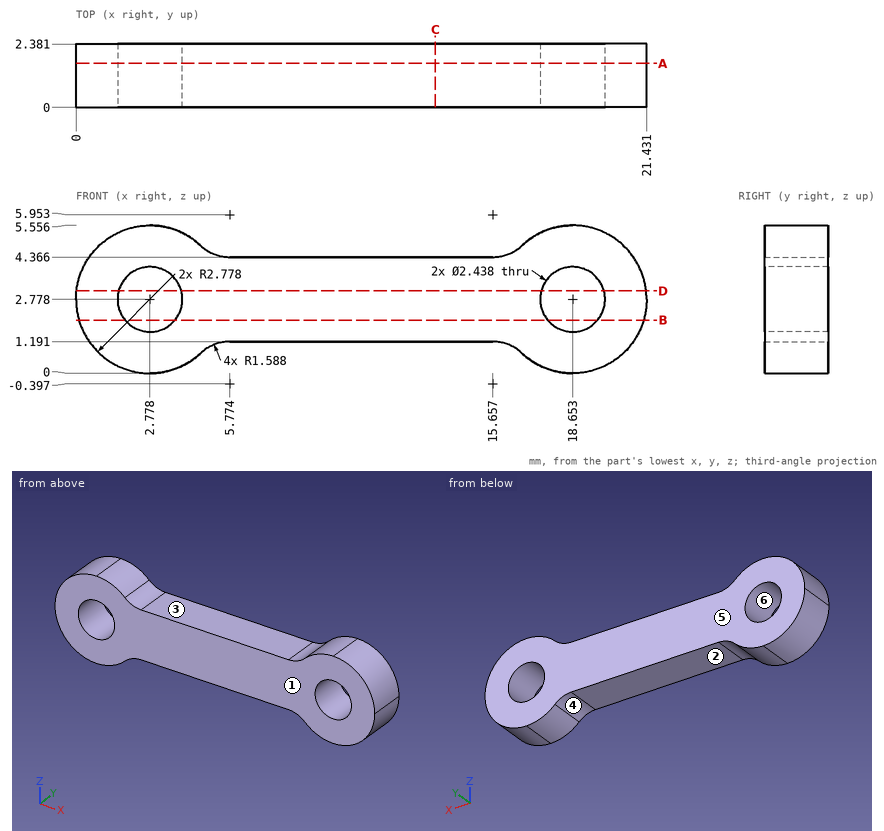
Source: three-view drawing plus pictorial views. Frame: mm from the lowest corner of the part. A direction names the side the tool comes from. Round coordinates to 2 decimals unless told otherwise and drop trailing zeros. Order: outer loops, then holes, each group sorted by start corner. A loop starts at its lowest first (then second) coordinate and runs counter-clockwise, first axis right, second up. Notation, with made-up numbers: M -39.75,-18.75 L 12.25,-18.75 A32 ccw 12.25,20.25 Z; hole C 50.5,-13 d1. An arc over 180 degrees is marked long. One line per item, written item: value.
(1) Cut plane C-C (x = 13.5). Return the cut outline in (y, z) (1 decimal).
Result sheet:
outline: M 0,1.2 L 2.4,1.2 L 2.4,4.4 L 0,4.4 Z
(2) Cut plane B-B (z = 2). Return the cut outline in (x, y) (1 decimal).
Result sheet:
outline: M 0.1,0 L 1.8,0 L 1.8,2.4 L 0.1,2.4 Z; M 3.7,0 L 17.7,0 L 17.7,2.4 L 3.7,2.4 Z; M 19.6,0 L 21.3,0 L 21.3,2.4 L 19.6,2.4 Z
(3) Pin query (flat end, axial travel): P1, Ø0.7, axis at x = 12.5, y = 1, coming from the -Z side; P2, Ø1.2, axis at x = 8.5, y = 1.5, coming from the +Z side. Return the tip coordinate at first contact, or that it passes through.
Result sheet:
P1: z = 1.19
P2: z = 4.37
(4) Pull-direction query (Z, two-part tool) for the marked faces 4, 5 and 6; classes: pulls with the +Z half, pulls with the -Z half, needs draft (parallel to the pull), parting line crosses it, or undercut.
Result sheet:
face 4: pulls with the -Z half
face 5: needs draft
face 6: undercut
(5) Reachability of the marked faces 1, 2 and 3 from +Z, -Z, +X, -X, +Y, -Y: full face, straight path, thin tool, end or side. Return the list, or none.
Result sheet:
face 1: +Z, -Z, +X, -X, -Y
face 2: -Z, +Y, -Y
face 3: +Z, +Y, -Y
(6) Line query: probe 1 along X at (y, z) = (0.25, 2.05) (1 decimal); probe 2 along Z at (x, y) = (13, 0.65) (1 decimal); probe 3 along X at (y, z) = (1.2, 2) (1 decimal). Output: solid intervals per line, ascending. Write a range as [from, to].
Result sheet:
probe 1: [0.1, 1.8], [3.8, 17.7], [19.6, 21.3]
probe 2: [1.2, 4.4]
probe 3: [0.1, 1.8], [3.7, 17.7], [19.6, 21.3]
(7) Cut plane A-A (y = 1.65). Give the number of separate pieces and of enclosed holes in the cut face.
Result sheet:
separate pieces: 1
enclosed holes: 2
(8) Cut plane D-D (z = 3.1). Return the cut outline in (x, y) (1 decimal).
Result sheet:
outline: M 0,0 L 1.6,0 L 1.6,2.4 L 0,2.4 Z; M 4,0 L 17.5,0 L 17.5,2.4 L 4,2.4 Z; M 19.8,0 L 21.4,0 L 21.4,2.4 L 19.8,2.4 Z
